The model under review builds one solid part; all positions refer to its coordinate system, in mm. A direction names the side the tool comes from. Give positions to 0.01 mm unless a question says otherwise; leave off trailing zeros. Order: outer loops, then holes, each group sorted by start corner. A loop starts at its lowest first (then second) coordinate and runs counter-clockwise, first axis right, second up. Notation, with made-up numbers: (86, -17.75) - (136, -17.75) arc R26 cw to (136, 14.25) - close; hole circle Ø10 at (-2, 46). An arc over 180 degrees is marked (long way). Write item = value, one per line. Start each with the question number.
1. We need section C-C, the plane x = -115.5. Give the boundary of the cut face in (y, z).
2. For P1, Ø1.5, axis at x = 90, z = 3.5, coming from the -Y side; P2, Ø1.5, axis at x = -104, z = -14.5, coming from the +Y side; P3, Ø8, axis at x = 67, y = -6.5, coming from the +Z side, all flat-tipped, find the tip position at first contact; note any pin that passes through.
3. Machinability: for faces 1 (the flat face through (139.7, 0, 0)), 2 (the flat face through (88, 0, -4.762)), which of the approach directions +Z, -Z, +X, -X, +Y, -Y give a long, thin tool a straight path to every point of the face, cutting with its end or side? Answer none if there is none.
4. We need section A-A, the plane z = 13.5. Give the boundary of the cut face in (x, y).
5. We need section B-B, the plane y = -8. Give the boundary of the cut face in (x, z) (1 decimal).
6. We need section D-D, the plane z = -8.5. Give the boundary of the cut face in (x, y), and give its area (3 significant figures).
7. Wall thickness on probe 1 along Z at (x, y) = (-110, 4); probe 2 along Y at (x, z) = (104, -1); probe 3 along Y at (x, z) = (-104.5, -16.5): over which ranges is each line inside the solid? List them lowest first.
8. Mouldability with a two-part tool opening along X and no side actions: class faces 3 (the flat face through (-12.482, 0.303, 10.793)), 4 (the flat face through (-67.328, 0.265, -14.144)), 5 (the flat face through (-15, 0, -11.112)) as pulls with the +X half, pulls with the -X half, needs draft (parallel to the pull), parting line crosses it, or undercut.
from build123d import *

# Parameters (mm, degrees)
F1_DEPTH      = 139.7
F1_DEPTH_BACK = 139.7
F3_DEPTH      = 22.501
F3_DEPTH_BACK = 22.501
F5_DEPTH      = 22.501
F5_DEPTH_BACK = 22.501


with BuildPart() as f1:
    # F0 (on Right) → F1 (new body, two sides)
    with BuildSketch(Plane.YZ) as f1_sk:
        with BuildLine():
            ThreePointArc((-3.45, 19.05), (-22.5, 0), (-3.45, -19.05))
            Line((-3.45, -19.05), (3.45, -19.05))
            ThreePointArc((3.45, -19.05), (22.5, 0), (3.45, 19.05))
            Line((3.45, 19.05), (-3.45, 19.05))
        make_face()
    extrude(amount=F1_DEPTH)
    extrude(f1_sk.sketch, amount=-F1_DEPTH_BACK)

    # F2 (on Front) → F3 (cut, two sides)
    with BuildSketch(Plane.XZ) as f3_sk:
        Polygon((139.7, 19.05), (-63.5, 19.05), (-61.6669128953, 15.875), (38.1, 5.5668172272), (32.1485679013, 15.875), (139.7, 4.7625), align=None)
    extrude(amount=-F3_DEPTH, mode=Mode.SUBTRACT)
    extrude(f3_sk.sketch, amount=F3_DEPTH_BACK, mode=Mode.SUBTRACT)

    # F4 (on Front) → F5 (cut, two sides)
    with BuildSketch(Plane.XZ) as f5_sk:
        Polygon((139.7, -19.05), (139.7, -4.7625), (35.4805530134, -4.7625), (34.925, -11.1125), (-67.0630954944, -11.1125), (-67.7575367611, -19.05), align=None)
    extrude(amount=-F5_DEPTH, mode=Mode.SUBTRACT)
    extrude(f5_sk.sketch, amount=F5_DEPTH_BACK, mode=Mode.SUBTRACT)


solid = f1.part
Model answer:
q1.outline = (-3.45, -19.05) - (3.45, -19.05) arc R19.05 ccw to (3.45, 19.05) - (-3.45, 19.05) arc R19.05 ccw to start
q2.P1 = -22.3
q2.P2 = 16.63
q2.P3 = 12.69
q3.face_1 = +Z, -Z, +X, +Y, -Y
q3.face_2 = -Z, +X, +Y, -Y
q4.outline = (-139.7, -16.89) - (-38.68, -16.89) - (-38.68, 16.89) - (-139.7, 16.89) - close; (33.52, -16.89) - (55.13, -16.89) - (55.13, 16.89) - (33.52, 16.89) - close
q5.outline = (-139.7, -18.5) - (-67.7, -18.5) - (-67.1, -11.1) - (34.9, -11.1) - (35.5, -4.8) - (139.7, -4.8) - (139.7, 4.8) - (32.1, 15.9) - (38.1, 5.6) - (-61.7, 15.9) - (-63.2, 18.5) - (-139.7, 18.5) - close
q6.outline = (-139.7, -20.5) - (35.15, -20.5) - (35.15, 20.5) - (-139.7, 20.5) - close
q6.area = 7,170 mm2
q7.probe_1 = -19.04 to 19.04
q7.probe_2 = -22.47 to 22.47
q7.probe_3 = -12.97 to 12.97
q8.face_3 = undercut
q8.face_4 = pulls with the +X half
q8.face_5 = needs draft
